Could you check a few things on this model? Use its own coordinates, in mm. Round coordinates to 2 decimals unless told otherwise and drop trailing zeros. Loops run counter-clockwise (first coordinate to the right, second up) from the corner with the lowest first, then second, coordinate; pieces in that order, holes last. Notation, with made-up numbers: (-32, 36) -> (9, 36) arc R22 ccw to (9, 75) -> close; hole circle Ø10 at (71, 84.5). An arc over 180 degrees is marked (long way). Put each result on its own line as item: value. Start each with the question number.
1. I need wall thicknesses on line 1 (X direction, y = -1, z = 51); line 2 (Z direction, x = -18, y = -9.5); line 3 (X direction, y = 26, z = 39.5). Which ranges of each line are inside material? Lowest first, please. Write a range as [from, to].
2. Imagine slicing it at A-A, the plane z = 21.5. Please give me the cut outline in (x, y).
3. Imagine slicing it at B-B, the plane x = -19. Please give me the cut outline in (y, z) (3 decimals), and give its area (3 significant figures).
4. Imagine slicing it at D-D, the plane y = -14.5. Please give me the cut outline in (x, z).
5. I'm going to push flat-ended pins straight in: P1, Ø10, axis at x = -21.5, y = -10.5, coming from the +Z side; P2, Ø10, axis at x = -2.5, y = 21.5, coming from the +Z side; P3, Ø5, axis at x = -7, z = 35, coming from the +Y side. Where does each tip first touch, or does it pass through?
6. Imagine slicing it at C-C, the plane y = 11.5. Please give me the cut outline in (x, z).
```python
from build123d import *

# Parameters (mm, degrees)
BOSS_EXTRUDE1_DEPTH     = 60
CUT_EXTRUDE1_DEPTH      = 60
CUT_EXTRUDE1_DEPTH_BACK = 60


with BuildPart() as part:
    # Sketch1 → Boss-Extrude1 (new body)
    with BuildSketch(Plane.XY):
        with BuildLine():
            Line((-30, 0), (-20, 10))
            ThreePointArc((-20, 10), (0, 30), (20, 10))
            Line((20, 10), (30, 0))
            ThreePointArc((30, 0), (0, -30), (-30, 0))
        make_face()
    extrude(amount=BOSS_EXTRUDE1_DEPTH)

    # Sketch2 → Cut-Extrude1 (cut, two sides)
    with BuildSketch(Plane(origin=(0, 0, 0), x_dir=(0, 0, -1), z_dir=(1, 0, 0))) as cut_extrude1_sk:
        with BuildLine():
            Line((-10, 10), (0, 0))
            Line((0, 0), (0, 30))
            Line((0, 30), (-30, 30))
            ThreePointArc((-30, 30), (-15.857864376, 24.142135624), (-10, 10))
        make_face()
        with BuildLine():
            ThreePointArc((-50, 10), (-44.142135624, 24.142135624), (-30, 30))
            Line((-30, 30), (-60, 30))
            Line((-60, 30), (-60, 0))
            Line((-60, 0), (-50, 10))
        make_face()
        with BuildLine():
            Line((-60, -30), (-30, -30))
            ThreePointArc((-30, -30), (-51.213203436, -21.213203436), (-60, 0))
            Line((-60, 0), (-60, -30))
        make_face()
        with BuildLine():
            Line((0, -30), (0, 0))
            ThreePointArc((0, 0), (-8.786796564, -21.213203436), (-30, -30))
            Line((-30, -30), (0, -30))
        make_face()
    extrude(amount=CUT_EXTRUDE1_DEPTH, mode=Mode.SUBTRACT)
    extrude(cut_extrude1_sk.sketch, amount=-CUT_EXTRUDE1_DEPTH_BACK, mode=Mode.SUBTRACT)


solid = part.part
```
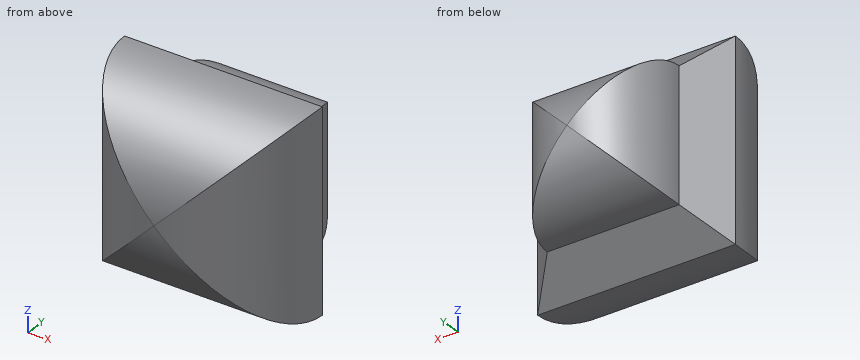
Entries:
1. line 1: [-29.98, 29.98]
1. line 2: [1.54, 58.46]
1. line 3: [-12, 12]
2. outline: (-30, 0) arc R30 ccw to (-8.5, -28.77) -> (8.5, -28.77) arc R30 ccw to (30, 0) -> (20, 10) arc R20 ccw to (8.5, 28.1) -> (-8.5, 28.1) arc R20 ccw to (-20, 10) -> close
3. outline: (-23.216, 11) arc R30 ccw to (0, 0) -> (10, 10) arc R20 ccw to (16.245, 11) -> (16.245, 49) arc R20 ccw to (10, 50) -> (0, 60) arc R30 ccw to (-23.216, 49) -> close
3. area: 1,980 mm^2
4. outline: (-26.26, 3.74) -> (26.26, 3.74) -> (26.26, 56.26) -> (-26.26, 56.26) -> close
5. P1: z = 59.49
5. P2: z = 48.91
5. P3: y = 29.48
6. outline: (-19.94, 10.06) -> (19.94, 10.06) -> (19.94, 49.94) -> (-19.94, 49.94) -> close
